Read the model definition and answer for the solid it produces. Units are mm, in the model's axes. Face numbers are marked on the shaded views. A direction names the side the tool comes from. Coordinates: 2 decimals unless noted, no trailing zeros. Order: outer loops, then holes, each group sorted by start corner. A loop starts at its lowest first (then second) coordinate and runs counter-clockwise, first axis right, second up. Notation, with made-up numbers: (-8, -38.75) -> (-1, -38.75) arc R11 ccw to (-1, -25.75) -> close; hole circle Ø9 at (46.25, 27.5). An arc over 180 degrees is marked (long way). Return JSON: item names as keys, results as strings. Group by question number.
```python
from build123d import *

# Parameters (mm, degrees)
SKETCH1_W                                           = 10
SKETCH1_H                                           = 10
BOSS_EXTRUDE1_DEPTH                                 = 133
SKETCH3_W                                           = 1.8
SKETCH3_H                                           = 120
CUT_EXTRUDE1_DEPTH                                  = 5
FILLET1_R                                           = 0.9
SKETCH4_W                                           = 10
SKETCH4_H                                           = 10
BOSS_EXTRUDE3_DEPTH                                 = 15
CBORE_FOR_M3_HEX_SOCKET_HEAD_CAP_SCREW1_D           = 3.4
CBORE_FOR_M3_HEX_SOCKET_HEAD_CAP_SCREW1_CBORE_D     = 6.5
CBORE_FOR_M3_HEX_SOCKET_HEAD_CAP_SCREW1_CBORE_DEPTH = 3.4
F_1_0MM_DOWEL_HOLE1_D                               = 1
F_1_0MM_DOWEL_HOLE1_DEPTH                           = 8
F_1_0MM_DOWEL_HOLE1_TIP                             = 0.30043031


with BuildPart() as part:
    # Sketch1 → Boss-Extrude1 (new body)
    with BuildSketch(Plane(origin=(0, 0, 0), x_dir=(1, 0, 0), z_dir=(0, 1, 0))):
        Rectangle(SKETCH1_W, SKETCH1_H)
    extrude(amount=BOSS_EXTRUDE1_DEPTH)

    # Sketch3 → Cut-Extrude1 (cut)
    with BuildSketch(Plane(origin=(5, 0, 0), x_dir=(0, 0, -1), z_dir=(1, 0, 0))):
        with Locations((0, 73)):
            Rectangle(SKETCH3_W, SKETCH3_H)
    extrude(amount=-CUT_EXTRUDE1_DEPTH, mode=Mode.SUBTRACT)

    # Fillet1
    fillet1_edges = [part.edges().sort_by_distance(p)[0] for p in [
        (2.5, 13, 0.9),
        (2.5, 13, -0.9),
    ]]
    fillet(fillet1_edges, radius=FILLET1_R - 0.0001)  # a hair under: the kernel refuses the full size

    # Sketch4 → Boss-Extrude3 (add, symmetric)
    with BuildSketch(Plane(origin=(0, 0, 0), x_dir=(0, 0, -1), z_dir=(1, 0, 0))):
        with Locations((0, 5)):
            Rectangle(SKETCH4_W, SKETCH4_H)
    extrude(amount=BOSS_EXTRUDE3_DEPTH, both=True)

    # CBORE for M3 Hex Socket Head Cap Screw1 (through all)
    with Locations(Plane(origin=(10, 10, 0), x_dir=(0, 0, 1), z_dir=(0, 1, 0))):
        with Locations((0, 0)):
            cbore_for_m3_hex_socket_head_cap_screw1 = CounterBoreHole(CBORE_FOR_M3_HEX_SOCKET_HEAD_CAP_SCREW1_D / 2, CBORE_FOR_M3_HEX_SOCKET_HEAD_CAP_SCREW1_CBORE_D / 2, CBORE_FOR_M3_HEX_SOCKET_HEAD_CAP_SCREW1_CBORE_DEPTH)

    # Mirror1: CBORE for M3 Hex Socket Head Cap Screw1 across plane
    add(cbore_for_m3_hex_socket_head_cap_screw1.mirror(Plane(origin=(0, 0, 0), x_dir=(0, 0, 1), z_dir=(1, 0, 0))), mode=Mode.SUBTRACT)

    # Ø1.0mm Dowel Hole1
    with Locations(Plane(origin=(0, 0, 0), x_dir=(0, 0, -1), z_dir=(0, -1, 0))):
        with Locations((0, 0)):
            Hole(F_1_0MM_DOWEL_HOLE1_D / 2, depth=F_1_0MM_DOWEL_HOLE1_DEPTH)
            with Locations((0, 0, -(F_1_0MM_DOWEL_HOLE1_DEPTH + F_1_0MM_DOWEL_HOLE1_TIP / 2))):  # 118° drill point
                Cone(0, F_1_0MM_DOWEL_HOLE1_D / 2, F_1_0MM_DOWEL_HOLE1_TIP, mode=Mode.SUBTRACT)


solid = part.part
```
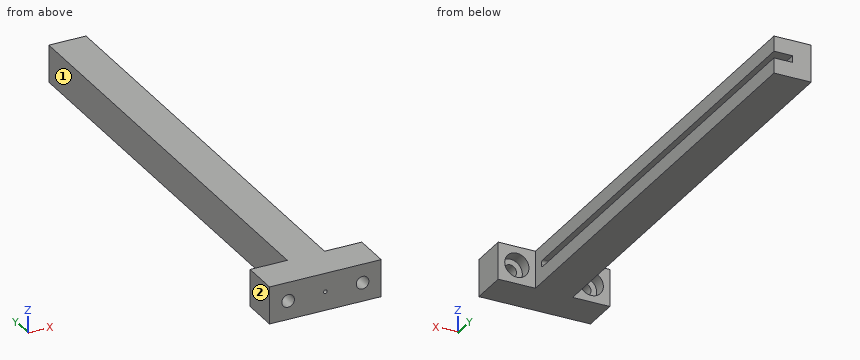
1. Given pin 1 (1.5 mm diameter, centred on y = 41.5, z = 3, fed in from -X); pin 2 (4 mm diameter, centred on x = -11, z = 3.5, fed in from +Y); pin 3 (2.5 mm diameter, centred on x = -10, z = 0, fed in from -Y); pin 4 (3 mm diameter, centred on x = -10.5, z = 1, fed in from +Y), each flat-ended and moving along its own axis, determine where each tip first touches the part or whether it passes through.
2. Which of the six approach directions +Z, -Z, +X, -X, +Y, -Y give full straight-line access (tool end or side, diameter ignored) to the marked faces 1 and 2?
3. Find section A-A on x = 10. Determine the outline of the cut face in (y, z).
4. Find section B-B on y = 115.5. Determine the outline of the cut face in (x, z).
5. Straight lines are drawn through the part: L1, parallel to X at y = 8.35, z = 0; L2, parallel to X at y = 4.5, z = 0; L3, parallel to Z at x = 0, y = 6. For each, find the intervals that lie inside material, in ascending order.
Result:
{
 "1": {"pin 1": "x = -5", "pin 2": "y = 10", "pin 3": "through", "pin 4": "y = 6.6"},
 "2": {"face 1": "+Z, -Z, -X, +Y", "face 2": "+Z, -Z, -X, +Y, -Y"},
 "3": {"outline": "(0, -5) -> (10, -5) -> (10, -3.25) -> (6.6, -3.25) -> (6.6, -1.7) -> (0, -1.7) -> close; (0, 1.7) -> (6.6, 1.7) -> (6.6, 3.25) -> (10, 3.25) -> (10, 5) -> (0, 5) -> close"},
 "4": {"outline": "(-5, -5) -> (5, -5) -> (5, -0.9) -> (0, -0.9) -> (0, 0.9) -> (5, 0.9) -> (5, 5) -> (-5, 5) -> close"},
 "5": {"L1": "-15 to -13.25, -6.75 to 6.75, 13.25 to 15", "L2": "-15 to -11.7, -8.3 to -0.5, 0.5 to 8.3, 11.7 to 15", "L3": "-5 to -0.5, 0.5 to 5"}
}
